from build123d import *

# Parameters (mm, degrees)
SALIENTE_EXTRUIR1_DEPTH = 20


with BuildPart() as part:
    # Croquis1 → Saliente-Extruir1 (new body)
    with BuildSketch(Plane.XY):
        with BuildLine():
            ThreePointArc((34, 0), (24.04163056, 24.04163056), (0, 34))
            ThreePointArc((0, 34), (-24.04163056, -24.04163056), (34, 0))
        make_face()
        with BuildLine():
            Line((-2.5, 31), (0, 31))
            Line((0, 31), (2.5, 31))
            Line((2.5, 31), (2.5, 28.892040426))
            ThreePointArc((2.5, 28.892040426), (21.371710273, 19.602295784), (29, 0))
            ThreePointArc((29, 0), (28.309591911, -6.290230985), (26.271240976, -12.280956704))
            Line((26.271240976, -12.280956704), (28.096787517, -13.334936491))
            Line((28.096787517, -13.334936491), (25.596787517, -17.665063509))
            Line((25.596787517, -17.665063509), (23.771240976, -16.611083723))
            ThreePointArc((23.771240976, -16.611083723), (0, -29), (-23.771240976, -16.611083723))
            Line((-23.771240976, -16.611083723), (-25.596787517, -17.665063509))
            Line((-25.596787517, -17.665063509), (-28.096787517, -13.334936491))
            Line((-28.096787517, -13.334936491), (-26.271240976, -12.280956704))
            ThreePointArc((-26.271240976, -12.280956704), (-25.11473671, 14.5), (-2.5, 28.892040426))
            Line((-2.5, 28.892040426), (-2.5, 31))
        make_face(mode=Mode.SUBTRACT)
    extrude(amount=SALIENTE_EXTRUIR1_DEPTH)


solid = part.part
Could you check a few things on this model? Use its own coordinates, in mm. A direction names the side the tool comes from. Round coordinates to 2 decimals unless told otherwise and drop trailing zeros. Loops run counter-clockwise (first coordinate to the right, second up) from the corner with the lowest first, then second, coordinate; pieces in that order, holes last. Notation, with made-up numbers: (79.25, 8.25) -> (112.25, 8.25) arc R34 ccw to (112.25, 38.25) -> close; hole circle Ø3 at (66, -26). An arc over 180 degrees is marked (long way). Use CSV: the item, a comma, the result in double quotes.
(1) If I drill on probe 1 along Y at (x, z) = (1, 10.5); probe 2 along X at (y, z) = (-1, 9.75); probe 3 along X at (y, z) = (14.5, 17.25), over which ranges is the centre line in solid material (lowest first)? Write a range as [from, to].
Return value:
probe 1,"y = [-33.99, -28.98], [31, 33.99]"
probe 2,"x = [-33.99, -28.98], [28.98, 33.99]"
probe 3,"x = [-30.75, -25.11], [25.11, 30.75]"
(2) For faces 3 (the flat face through (-2.5, 30, 10)), 4 (the flat face through (28, 10, 0)), which set-ups out of +Z, -Z, +X, -X, +Y, -Y let a thin tool reach every point of the face, with its end or its side?
Return value:
face 3,"+Z, -Z"
face 4,"-Z, +X, -X, +Y, -Y"
(3) Suppose I cut it at A-A on x = 16.5. Write out the boundary of the cut face in (y, z), plus the area to 3 significant figures.
Return value:
outline,"(-29.73, 0) -> (-23.85, 0) -> (-23.85, 20) -> (-29.73, 20) -> close; (23.85, 0) -> (29.73, 0) -> (29.73, 20) -> (23.85, 20) -> close"
area,"235 mm²"
(4) Will these pins go through, and if not, where does the flat tip stop? pin 1 Ø1.1 at (y, z) = (29.5, 7.5) entering from -X; pin 2 Ø1.5 at (x, z) = (-15.5, 17.5) entering from +Y; pin 3 Ø4 at (y, z) = (22, 15.5) entering from -X; pin 4 Ø8 at (x, y) = (5, 22) entering from -Z.
Return value:
pin 1,"stops at x = -17.83"
pin 2,"stops at y = 30.63"
pin 3,"stops at x = -27.5"
pin 4,"passes through"
(5) If we mould it in two halves opening along X, with no side actions, what happens to faces 1 (the flat face through (28, 10, 20)), 2 (the flat face through (-26.83, -15.53, 9.86))? For each: +X half, -X half, draft (parallel to the pull), parting line (faces both ways), or undercut.
Return value:
face 1,"draft"
face 2,"undercut"
(6) Suppose I cut it at C-C on z = 5.75. Write out the boundary of the cut face in (x, y).
Return value:
outline,"circle Ø68 at (0, 0); hole (-28.1, -13.33) -> (-25.6, -17.67) -> (-23.77, -16.61) arc R29 ccw to (23.77, -16.61) -> (25.6, -17.67) -> (28.1, -13.33) -> (26.27, -12.28) arc R29 ccw to (2.5, 28.89) -> (2.5, 31) -> (-2.5, 31) -> (-2.5, 28.89) arc R29 ccw to (-26.27, -12.28) -> close"
(7) Suppose I cut it at B-B on y = 19.5. Write out the boundary of the cut face in (x, z), plus the area to 3 significant figures.
Return value:
outline,"(-27.85, 0) -> (-21.47, 0) -> (-21.47, 20) -> (-27.85, 20) -> close; (21.47, 0) -> (27.85, 0) -> (27.85, 20) -> (21.47, 20) -> close"
area,"255 mm²"
